Build history of the part. All positions in model axes, mm. A direction names the side the tool comes from. Give positions to 0.01 mm unless a question says otherwise; leave off trailing zeros. Write each loop counter-clockwise with the first axis right and the second up, starting at its lowest first coordinate (ties: lowest second). Pieces come first, ordered by that corner, then holes.
from build123d import *

# Parameters (mm, degrees)
F1_DEPTH = 3.429
F3_DEPTH = 457.2
F4_R     = 50.8
F5_DEPTH = 25.4


with BuildPart() as f1:
    # F0 (on Right) → F1 (new body)
    with BuildSketch(Plane.YZ):
        Polygon((-304.8, 0), (0, 0), (0, 457.2), align=None)
    extrude(amount=F1_DEPTH)

    # F2 (on Top) → F3 (join, through all)
    with BuildSketch(Plane.XY):
        Polygon((0, 38.1), (0, 0), (3.429, 0), (3.429, 41.529), (-41.021, 41.529), (-41.021, 38.1), align=None)
    extrude(amount=F3_DEPTH)

    # F4 (on face) → F5 (cut)
    with BuildSketch(Plane.YZ.offset(3.429)):
        with Locations((-136.271, 0)):
            Circle(F4_R)
    extrude(amount=-F5_DEPTH, mode=Mode.SUBTRACT)


solid = f1.part
(1) Saw through at A-A, the plane z = 36. List the corners of the cut face in (x, y), plus the area to 3 significant figures.
(2) Drop flat-ended pins along their axis: pin 1 (1.5 mm diameter, centred on x = -30, z = 379.5, fed in from -Y); pin 2 (1.5 mm diameter, centred on y = -25, z = 308.5, fed in from -X). Give the stop position or say it passes through.
(3) Saw through at B-B, the plane z = 231. List the corners of the cut face in (x, y).
(4) 3-axis set-ups, long thin cutter, end or side, ignore diameter. For faces 1 (the face through (-21, 38.1, 225)), 2 (the face through (-9, 39, 457.2)): which of +Z, -Z, +X, -X, +Y, -Y reach the whole face in a straight line?
(5) Mould opens along Y. For faces 3 (the face through (1.739, -135.154, 50.788)), 4 (the face through (0, -93, 175)), 5 (the face through (1.69, -150.266, 231.8)), 6 (the face through (-18, 41.529, 225)) say: +Y half, -Y half, draft (parallel to the pull), parting line (faces both ways), or undercut.
(6) Saw through at D-D, the plane x = -21.5. List the corners of the cut face in (y, z), plus the area to 3 significant figures.
(7) Probe line 1 (Y direction, x = -15.5, z = 228); line 2 (X direction, y = -88, z = 70.5); line 3 (Z direction, x = 1.5, y = -97). List the from-to ranges inside material, lowest first.
(8) Saw through at C-C, the plane y = -234. List the corners of the cut face in (x, z), plus the area to 3 significant figures.
Computed values:
1. outline: (-41.02, 38.1) - (0, 38.1) - (0, -100.43) - (3.43, -100.43) - (3.43, 41.53) - (-41.02, 41.53) - close; (0, -280.8) - (3.43, -280.8) - (3.43, -172.11) - (0, -172.11) - close
1. area: 1,000 mm2
2. pin 1: stops at y = 38.1
2. pin 2: stops at x = 0
3. outline: (-41.02, 38.1) - (0, 38.1) - (0, -150.8) - (3.43, -150.8) - (3.43, 41.53) - (-41.02, 41.53) - close
4. face 1: +Z, -Z, -X, -Y
4. face 2: +Z, +X, -X, +Y, -Y
5. face 3: undercut
5. face 4: draft
5. face 5: -Y half
5. face 6: +Y half
6. outline: (38.1, 0) - (41.53, 0) - (41.53, 457.2) - (38.1, 457.2) - close
6. area: 1,570 mm2
7. line 1: y = 38.1 to 41.53
7. line 2: x = 0 to 3.43
7. line 3: z = 32.22 to 311.7
8. outline: (0, 0) - (3.43, 0) - (3.43, 106.2) - (0, 106.2) - close
8. area: 364 mm2
